Geometry: final body of the model. Coordinates: model frame, mm. Face numbers are marked on the shaded views. A direction names the side the tool comes from. Give positions to 0.01 mm unless a question says otherwise; leave off trailing zeros. Write each loop counter-clockwise with the first axis right and the second up, starting at its lowest first coordinate (ties: lowest second). Pieces come first, ordered by that corner, then holes.
Q1. Line query: L1, parallel to X at y = -8, z = 4; L2, parallel to Z at x = 17, y = -1.5; L3, parallel to X at y = 17.5, z = 2.75. Output: solid intervals per line, ascending.
Q2. Cut plane C-C on y = -1. Return the cut outline in (x, z).
Q3. Cut plane A-A on z = 2. Return the cut outline in (x, y), plus the area to 3 significant figures.
Q4. Pin query (flat end, axial travel): pin 1 (4 mm diameter, centred on x = -10.95, y = -6.03, fed in from -Z); pin 2 (1.5 mm diameter, centred on y = -10.5, z = 11.5, fed in from +X); pin 3 (3 mm diameter, centred on x = 14.5, z = 1.5, fed in from +Y); pin 4 (6 mm diameter, centred on x = -10.95, y = -6.03, fed in from +Z). Return the tip coordinate at first contact, or that it passes through.
Q5. Draft query along X for the marked faces 5, 6 and 7. Return one class per face: pulls with the +X half, pulls with the -X half, needs draft (parallel to the pull), parting line crosses it, or undercut.
Q6. Reachability of the marked faces 1, 2, 3 and 4 from +Z, -Z, +X, -X, +Y, -Y: full face, straight path, thin tool, end or side. Return the list, or none.
Q7. Cut plane D-D on x = -15.5. Return the cut outline in (y, z), plus the area to 3 significant figures.
Q8. Cut plane B-B on z = 12. Return the cut outline in (x, y), plus the area to 3 significant figures.
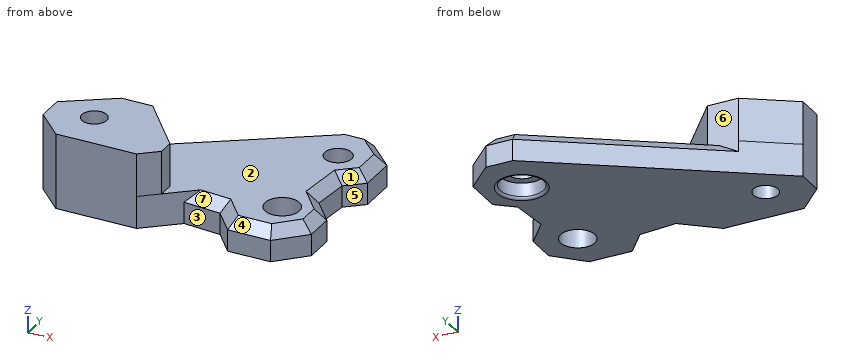
```python
from build123d import *

# Parameters (mm, degrees)
SKETCH_1_R          = 2.3
SKETCH_1_R_2        = 3.2
SKETCH_1_R_3        = 2.5
EXTRUDE_1_DEPTH     = 6
CHAMFER_1_SIZE      = 5
EXTRUDE_2_DEPTH     = 8
SKETCH_4_R          = 2.3
CUT_EXTRUDE_1_DEPTH = 8
CHAMFER_3_SIZE      = 2
SKETCH_5_R          = 4.05
CUT_EXTRUDE_2_DEPTH = 3
FILLET_1_R          = 0.5


with BuildPart() as part:
    # 草图1 → 凸台-拉伸1 (new body)
    with BuildSketch(Plane.XY):
        Polygon((21.045855827, 22.973933312), (-18.954144173, -4.026066688), (-18.954144173, -14.026066688), (1.045855827, -14.026066688), (11.078642712, -5.66541095), (18.045855827, -14.026066688), (31.045855827, -14.026066688), (31.045855827, -3.521043084), (23.917178911, 5.033369215), (31.045855827, 10.973933312), (31.045855827, 22.973933312), align=None)
        with Locations((-10.954144173, -6.026066688)):
            Circle(SKETCH_1_R, mode=Mode.SUBTRACT)
        with Locations((24.045855827, -6.026066688)):
            Circle(SKETCH_1_R_2, mode=Mode.SUBTRACT)
        with Locations((24.045855827, 13.973933312)):
            Circle(SKETCH_1_R_3, mode=Mode.SUBTRACT)
    extrude(amount=EXTRUDE_1_DEPTH)

    # 倒角1
    chamfer_1_edges = [part.edges().sort_by_distance(p)[0] for p in [
        (23.917178911, 5.033369215, 3),
        (31.045855827, -14.026066688, 3),
        (11.078642712, -5.66541095, 3),
        (-18.954144173, -14.026066688, 3),
        (31.045855827, 22.973933312, 3),
    ]]
    chamfer(chamfer_1_edges, length=CHAMFER_1_SIZE)

    # 草图3 → 凸台-拉伸2 (add)
    with BuildSketch(Plane.XY.offset(6)):
        Polygon((-10.05036615, 1.983983477), (-4.262738325, 1.983983477), (4.318113554, -8.313038778), (4.318113554, -11.299185249), (1.045855827, -14.026066688), (-13.954144173, -14.026066688), (-18.954144173, -9.026066688), (-18.954144173, -4.026066688), align=None)
    extrude(amount=EXTRUDE_2_DEPTH)

    # 草图4 → 切除-拉伸1 (cut)
    with BuildSketch(Plane(origin=(0, 0, 6), x_dir=(-1, 0, 0), z_dir=(0, 0, -1))):
        with Locations((10.954144173, -6.026066688)):
            Circle(SKETCH_4_R)
    extrude(amount=-CUT_EXTRUDE_1_DEPTH, mode=Mode.SUBTRACT)

    # 倒角3
    chamfer_3_edges = [part.edges().sort_by_distance(p)[0] for p in [
        (10.758550512, -9.186425149, 6),
        (16.162710269, -11.766292018, 6),
        (22.045855827, -14.026066688, 6),
        (28.545855827, -11.526066688, 6),
        (31.045855827, -6.273554886, 6),
        (29.081978368, -1.164390133, 6),
        (27.438193109, 4.713277016, 6),
        (5.497744838, 12.478958395, 6),
        (23.545855827, 22.973933312, 6),
        (28.545855827, 20.473933312, 6),
        (31.045855827, 14.473933312, 6),
        (29.402070568, 9.604112263, 6),
    ]]
    chamfer(chamfer_3_edges, length=CHAMFER_3_SIZE)

    # 草图5 → 切除-拉伸2 (cut)
    with BuildSketch(Plane(origin=(0, 0, 0), x_dir=(-1, 0, 0), z_dir=(0, 0, -1))):
        with Locations((-24.045855827, 13.973933312)):
            Circle(SKETCH_5_R)
    extrude(amount=-CUT_EXTRUDE_2_DEPTH, mode=Mode.SUBTRACT)

    # 圆角1
    fillet_1_edges = [part.edges().sort_by_distance(p)[0] for p in [
        (28.095855827, 13.973933312, 0),
    ]]
    fillet(fillet_1_edges, radius=FILLET_1_R)


solid = part.part
```
Data:
1. L1: x = -18.95 to -12.13, -9.77 to 21.53, 26.56 to 31.05
1. L2: z = 0 to 6
1. L3: x = 12.94 to 22.05, 26.04 to 31.05
2. outline: (-14.47, 0) - (28.94, 0) - (28.94, 4) - (26.34, 6) - (-1.78, 6) - (-1.78, 14) - (-14.47, 14) - close
3. outline: (-18.95, -9.03) - (-13.95, -14.03) - (1.05, -14.03) - (7.24, -8.87) - (14.28, -9.51) - (18.05, -14.03) - (26.05, -14.03) - (31.05, -9.03) - (31.05, -3.52) - (27.12, 1.19) - (27.76, 8.23) - (31.05, 10.97) - (31.05, 17.97) - (26.05, 22.97) - (21.05, 22.97) - (-18.95, -4.03) - close; hole circle Ø4.6 at (-10.95, -6.03); hole circle Ø8.1 at (24.05, 13.97); hole circle Ø6.4 at (24.05, -6.03)
3. area: 1,070 mm2
4. pin 1: passes through
4. pin 2: stops at x = 4.32
4. pin 3: stops at y = 19.57
4. pin 4: stops at z = 14
5. face 5: pulls with the +X half
5. face 6: needs draft
5. face 7: undercut
6. face 1: +Z, +X
6. face 2: +Z, +X, +Y
6. face 3: +Z, -Z, -Y
6. face 4: +Z, +X, -Y
7. outline: (-12.48, 0) - (-1.69, 0) - (-1.69, 14) - (-12.48, 14) - close
7. area: 151 mm2
8. outline: (-18.95, -9.03) - (-13.95, -14.03) - (1.05, -14.03) - (4.32, -11.3) - (4.32, -8.31) - (-4.26, 1.98) - (-10.05, 1.98) - (-18.95, -4.03) - close; hole circle Ø4.6 at (-10.95, -6.03)
8. area: 268 mm2
